from build123d import *

# Parameters (mm, degrees)
SALIENTE_EXTRUIR1_DEPTH    = 30
CROQUIS2_W                 = 18
CROQUIS2_H                 = 35
CORTAR_EXTRUIR1_DEPTH      = 110.658560997
CROQUIS3_R                 = 20
SALIENTE_EXTRUIR2_DEPTH    = 22
CORTAR_EXTRUIR2_DEPTH      = 89.459030065
CORTAR_EXTRUIR2_DEPTH_BACK = 89.459030065
CROQUIS3_3_R               = 8
CROQUIS4_W                 = 24
CROQUIS4_H                 = 17
CORTAR_EXTRUIR4_DEPTH      = 15


with BuildPart() as part:
    # Croquis1 → Saliente-Extruir1 (new, symmetric)
    with BuildSketch(Plane(origin=(0, 0, 0), x_dir=(0, 0, -1), z_dir=(1, 0, 0))):
        Polygon((45, 0), (-45, 0), (-25, 55), (25, 55), align=None)
    extrude(amount=SALIENTE_EXTRUIR1_DEPTH, both=True)

    # Croquis2 → Cortar-Extruir1 (cut, through all)
    with BuildSketch(Plane.XY.offset(45)):
        with Locations((-21, 37.5)):
            Rectangle(CROQUIS2_W, CROQUIS2_H)
        with Locations((21, 37.5)):
            Rectangle(CROQUIS2_W, CROQUIS2_H)
    extrude(amount=-CORTAR_EXTRUIR1_DEPTH, mode=Mode.SUBTRACT)

    # Croquis3 → Saliente-Extruir2 (add, symmetric)
    with BuildSketch(Plane(origin=(0, 0, 0), x_dir=(0, 0, -1), z_dir=(1, 0, 0))):
        with Locations((0, 50)):
            Circle(CROQUIS3_R)
    extrude(amount=SALIENTE_EXTRUIR2_DEPTH, both=True)

    # Croquis3<3> → Cortar-Extruir2 (cut, two sides: drawn at the far end of the back side and taken through both)
    with BuildSketch(Plane(origin=(0, 0, 0), x_dir=(0, 0, -1), z_dir=(1, 0, 0)).offset(-CORTAR_EXTRUIR2_DEPTH_BACK)):
        with Locations((0, 50)):
            Circle(CROQUIS3_3_R)
    extrude(amount=CORTAR_EXTRUIR2_DEPTH + CORTAR_EXTRUIR2_DEPTH_BACK, mode=Mode.SUBTRACT)

    # Croquis4 → Cortar-Extruir4 (cut)
    with BuildSketch(Plane(origin=(0, 70, 0), x_dir=(1, 0, 0), z_dir=(0, 1, 0))):
        with Locations((0, -16.5)):
            Rectangle(CROQUIS4_W, CROQUIS4_H)
        with Locations((0, 16.5)):
            Rectangle(CROQUIS4_W, CROQUIS4_H)
    extrude(amount=-CORTAR_EXTRUIR4_DEPTH, mode=Mode.SUBTRACT)


solid = part.part
Here's how the part is built. I have some questions about the finished solid (model axes, mm). A direction names the side the tool comes from. Coordinates: 2 decimals unless noted, no trailing zeros. Order: outer loops, then holes, each group sorted by start corner. A loop starts at its lowest first (then second) coordinate and runs counter-clockwise, first axis right, second up. Notation, with made-up numbers: (-37.75, 76) - (-9.75, 76) arc R33 cw to (-9.75, 108) - close; hole circle Ø5 at (-26.5, 11.25). An arc over 180 degrees is marked (long way). Use CSV: the item, a comma, the result in double quotes. Start each with the question number.
1. Suppose I cut it at B-B on x = -5.5. List the corners of the cut face in (y, z) for me, then the cut area to 3 significant figures.
2. For faces 1 (the face through (-12, 29, 1)), 2 (the face through (12, 29, 1)), 3 (the face through (0.31, 69.83, 2.6)), 4 (the face through (21, 20, 1)), 5 (the face through (0, 62, 8)), which set-ups out of +Z, -Z, +X, -X, +Y, -Y let a thin tool reach every point of the face, with its end or its side?
3. Suppose I cut it at A-A on z = 0. List the corners of the cut face in (x, y) for me.
4. Suppose I cut it at C-C on y = 50. List the corners of the cut face in (x, z) for me, then the cut area to 3 significant figures.
5. Suppose I cut it at D-D on y = 11. List the corners of the cut face in (x, z) for me.
6. Please list where these lines run through material, in increasing order: line 1 (Y direction, x = -13, z = 0); line 2 (Y direction, x = -21, z = 2); line 3 (Z direction, x = 7.5, y = 60). Write a range as from..to.
7. If we mould it in two halves opening along X, with no side actions, what happens to faces 6 (the face through (-0.308, 57.932, 1.041)), 7 (the face through (0, 62, -8)), 8 (the face through (-30, 10, -1))? For each: +X half, -X half, draft (parallel to the pull), parting line (faces both ways), or undercut.
8. I'm going to push flat-ended pins straight in: pin 1 (4 mm diameter, centred on y = 34.5, z = -13.5, fed in from +X); pin 2 (17.5 mm diameter, centred on y = 34.5, z = 0.5, fed in from -X); pin 3 (8.5 mm diameter, centred on x = -4, z = 20, fed in from +Y). Where does each tip first touch, or does it pass through?
Output:
1,outline,"(0, -45) - (55, -25) - (55, -8) - (68.33, -8) arc R20 ccw to (68.33, 8) - (55, 8) - (55, 25) - (0, 45) - close; hole circle Ø16 at (50, 0)"
1,area,"3,880 mm2"
2,face 1,"-X"
2,face 2,"+X"
2,face 3,"none"
2,face 4,"+Z, -Z, +X"
2,face 5,"+Z, +Y"
3,outline,"(-30, 0) - (30, 0) - (30, 20) - (12, 20) - (12, 30) - (22, 30) - (22, 42) - (-22, 42) - (-22, 30) - (-12, 30) - (-12, 20) - (-30, 20) - close; (-22, 58) - (22, 58) - (22, 70) - (-22, 70) - close"
4,outline,"(-22, -20) - (-12, -20) - (-12, -26.82) - (12, -26.82) - (12, -20) - (22, -20) - (22, -8) - (-22, -8) - close; (-22, 8) - (22, 8) - (22, 20) - (12, 20) - (12, 26.82) - (-12, 26.82) - (-12, 20) - (-22, 20) - close"
4,area,"1,380 mm2"
5,outline,"(-30, -41) - (30, -41) - (30, 41) - (-30, 41) - close"
6,line 1,"y = 0..20, 30..42, 58..70"
6,line 2,"y = 0..20, 30.1..42.25, 57.75..69.9"
6,line 3,"z = -8..8"
7,face 6,"draft"
7,face 7,"undercut"
7,face 8,"-X half"
8,pin 1,"stops at x = 22"
8,pin 2,"stops at x = -22"
8,pin 3,"stops at y = 55"
